Could you check a few things on this model? Use its own coordinates, in mm. Coordinates: 2 decimals unless noted, no trailing zeros. Order: outer loops, then holes, each group sorted by start corner. A loop starts at its lowest first (then second) coordinate and runs counter-clockwise, first axis right, second up. Notation, with made-up numbers: (-33, 75) - (25, 75) arc R22 ccw to (25, 90) - close; hole circle Ø5 at (14, 50). An arc over 180 degrees is marked (long way). Answer as CSV lines item,"result". Start each with the question number.
1. I want a section at B-B, the plane z = 8.5. List the corners of the cut face in (x, y) for me, and give its area (4 significant figures).
2. I need wall thicknesses on probe 1 along Y at (x, z) = (24.5, 10); probe 2 along Y at (x, z) = (27, 8); probe 3 along X at (y, z) = (150, -8). Which ranges of each line are inside material? Lowest first, please.
3. For pin 1 (1.6 mm diameter, centred on x = 30.5, y = 28.5, fed in from -Z); pin 2 (2.5 mm diameter, centred on x = 28.5, z = -14.5, fed in from -Y); pin 3 (1.6 mm diameter, centred on x = 24, z = 21.5, fed in from +Y); pin 4 (8 mm diameter, centred on y = 39.5, z = -23.5, fed in from -X), each with a flat end and sliding along its axis, tell me the tip position at first contact or that it passes through.
4. I want a section at A-A, the plane y = 38.5. List the corners of the cut face in (x, z) for me, and give its area (3 significant figures).
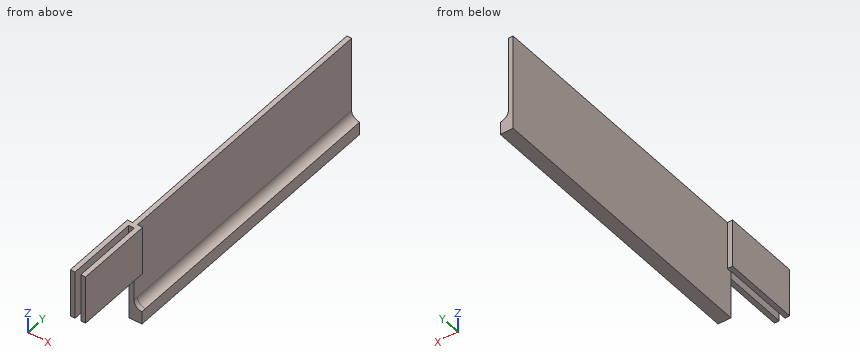
from build123d import *

# Parameters (mm, degrees)
SKETCH_1_W          = 3
SKETCH_1_H          = 45
EXTRUDE_1_DEPTH     = 30
EXTRUDE_1_2_DEPTH   = 30
SKETCH_2_W          = 9.5
SKETCH_2_H          = 30
EXTRUDE_2_DEPTH     = 3
SKETCH_3_W          = 3
SKETCH_3_H          = 60
EXTRUDE_3_DEPTH     = 180
SKETCH_4_W          = 5
SKETCH_4_H          = 8
EXTRUDE_4_DEPTH     = 180
FILLET_4_R          = 5
CUT_EXTRUDE_START   = -18
SKETCH_5_W          = 60.08866788
SKETCH_5_H          = 228
CUT_EXTRUDE_1_DEPTH = 11.25
EXTRUDE_5_DEPTH     = 3


with BuildPart() as part:
    # Sketch 1 → Extrude 1 (new body)
    with BuildSketch(Plane.XY):
        with Locations((1.5, 22.5)):
            Rectangle(SKETCH_1_W, SKETCH_1_H)
    extrude(amount=EXTRUDE_1_DEPTH)



with BuildPart() as body_2:
    # Sketch 1 → Extrude 1 2 (new body)
    with BuildSketch(Plane.XY):
        with Locations((8, 22.5)):
            Rectangle(SKETCH_1_W, SKETCH_1_H)
    extrude(amount=EXTRUDE_1_2_DEPTH)


with BuildPart() as part_1:
    add(part.part)

    add(body_2.part)  # Extrude 2 merges body 2
    # Sketch 2 → Extrude 2 (add)
    with BuildSketch(Plane(origin=(0, 45, 0), x_dir=(1, 0, 0), z_dir=(0, 1, 0))):
        with Locations((4.75, -15)):
            Rectangle(SKETCH_2_W, SKETCH_2_H)
    extrude(amount=EXTRUDE_2_DEPTH)

    # Sketch 3 → Extrude 3 (add)
    with BuildSketch(Plane(origin=(0, 48, 0), x_dir=(1, 0, 0), z_dir=(0, 1, 0))):
        with Locations((4.75, 0)):
            Rectangle(SKETCH_3_W, SKETCH_3_H)
    extrude(amount=EXTRUDE_3_DEPTH)

    # Sketch 4 → Extrude 4 (add)
    with BuildSketch(Plane(origin=(0, 228, 0), x_dir=(1, 0, 0), z_dir=(0, 1, 0))):
        with Locations((0.75, 26)):
            Rectangle(SKETCH_4_W, SKETCH_4_H)
    extrude(amount=-EXTRUDE_4_DEPTH)

    # Fillet 4
    fillet_4_edges = [part_1.edges().sort_by_distance(p)[0] for p in [
        (3.25, 138, -22),
    ]]
    fillet(fillet_4_edges, radius=FILLET_4_R - 0.0001)  # a hair under: the kernel refuses the full size


with BuildPart() as body_2_2:
    # Mirror 3: mirrored copy
    add(part_1.part.mirror(Plane(origin=(16.25, 0, 0), x_dir=(0, 0, 1), z_dir=(1, 0, 0))))

    # Sketch 6 → Extrude 5 (add)
    with BuildSketch(Plane.XZ.offset(-48)):
        with BuildLine():
            Line((26.25, 0), (26.25, -30))
            Line((26.25, -30), (34.25, -30))
            Line((34.25, -30), (34.25, -22))
            ThreePointArc((34.25, -22), (30.714466094, -20.535533906), (29.25, -17))
            Line((29.25, -17), (29.25, 0))
            Line((29.25, 0), (26.25, 0))
        make_face()
    extrude(amount=EXTRUDE_5_DEPTH)


with BuildPart() as part_2:
    add(part_1.part)

    # Sketch 5 → Cut-Extrude 1 (cut)
    with BuildSketch(Plane(origin=(16.25, 0, 0), x_dir=(0, 0, -1), z_dir=(1, 0, 0)).offset(CUT_EXTRUDE_START)):
        with Locations((0.04433394, 114)):
            Rectangle(SKETCH_5_W, SKETCH_5_H)
    extrude(amount=CUT_EXTRUDE_1_DEPTH, mode=Mode.SUBTRACT)


solid = body_2_2.part
Solved:
1,outline,"(23, 0) - (26, 0) - (26, 45) - (29.5, 45) - (29.5, 0) - (32.5, 0) - (32.5, 48) - (29.25, 48) - (29.25, 228) - (26.25, 228) - (26.25, 48) - (23, 48) - close"
1,area,"838.5 mm2"
2,probe 1,"y = 0 to 48"
2,probe 2,"y = 45 to 228"
2,probe 3,"x = 26.25 to 29.25"
3,pin 1,"stops at z = 0"
3,pin 2,"stops at y = 45"
3,pin 3,"stops at y = 48"
3,pin 4,"passes through"
4,outline,"(23, 0) - (26, 0) - (26, 30) - (23, 30) - close; (29.5, 0) - (32.5, 0) - (32.5, 30) - (29.5, 30) - close"
4,area,"180 mm2"
